The drawing under review shows one solid part. Ordinate dimensions are in mm from its lowest x, y, z. A direction names the side the tool comes from. Coordinates: 2 decimals unless noted, no trailing zeros. Write each loop counter-clockwise with the first axis right and the second up, starting at its lowest first coordinate (ties: lowest second). Pieces come first, ordered by that corner, then holes.
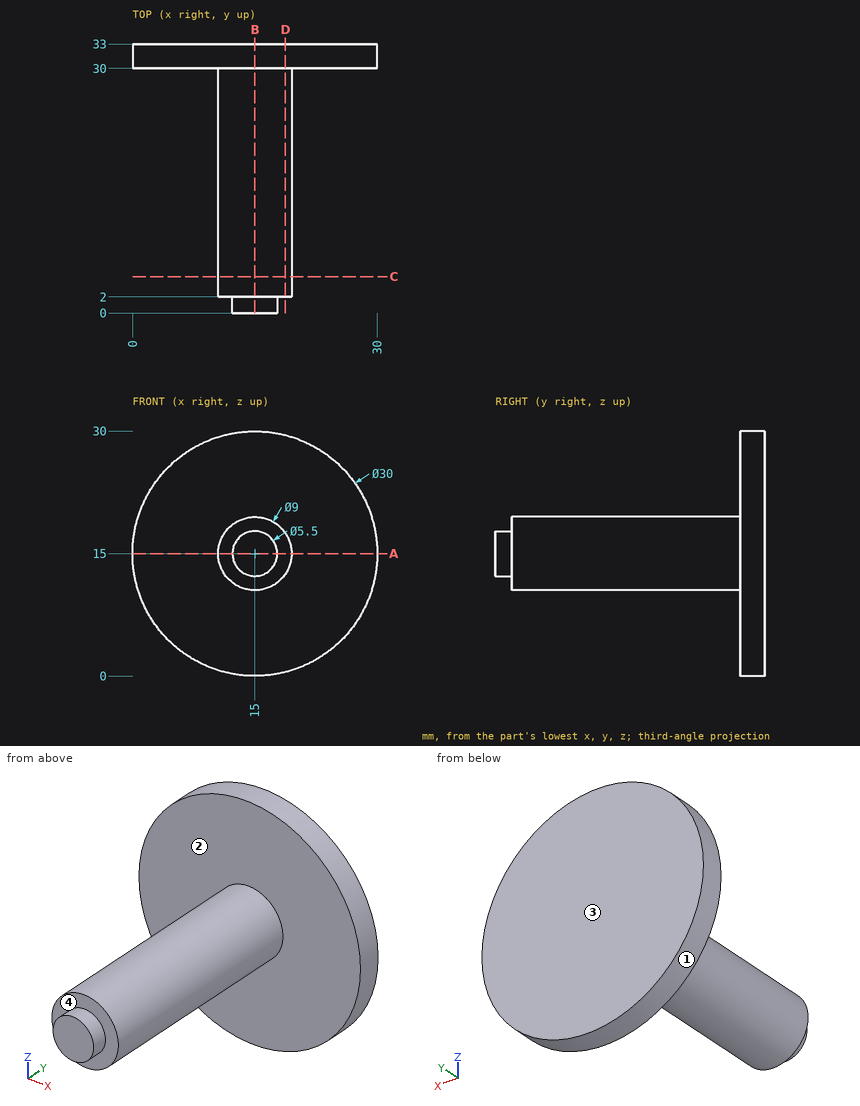
Q1. Draft analysis for pull direction Z (two halves, no side actions). For the marked faces 1 and 2, state which applies: +Z half, -Z half, draft (parallel to the pull), parting line (faces both ways), or undercut.
Ans:
face 1: parting line
face 2: draft
Q2. Add section D-D (x = 18.75). State the section outline as (y, z) points, then the cut area to 3 significant figures.
Ans:
outline: (2, 12.51) - (30, 12.51) - (30, 0.48) - (33, 0.48) - (33, 29.52) - (30, 29.52) - (30, 17.49) - (2, 17.49) - close
area: 226 mm2
Q3. Add section C-C (y = 4.5). State the section outline as (x, z) points.
Ans:
outline: circle Ø9 at (15, 15)
Q4. Add section A-A (z = 15). State the section outline as (x, y) points.
Ans:
outline: (0, 30) - (10.5, 30) - (10.5, 2) - (12.25, 2) - (12.25, 0) - (17.75, 0) - (17.75, 2) - (19.5, 2) - (19.5, 30) - (30, 30) - (30, 33) - (0, 33) - close
Q5. Clearance check with flat-ended pins moving along their axes: pin 1 Ø2 at (x, z) = (17, 22.5) entering from -Y; pin 2 Ø10 at (y, z) = (16, 11) entering from -X; pin 3 Ø10 at (x, y) = (20, 15.5) entering from +Z; pin 4 Ø2 at (x, y) = (9, 13.5) entering from -Z. State where each tip first meets the part, or that it passes through.
Ans:
pin 1: stops at y = 30
pin 2: stops at x = 10.5
pin 3: stops at z = 19.5
pin 4: passes through
Q6. Tool access review of the marked faces 3 and 4: name each direction out of +Z, -Z, +X, -X, +Y, -Y from which nothing blocks a thin tool from reaching the whole face with its end or side.
Ans:
face 3: +Z, -Z, +X, -X, +Y
face 4: -Y
Q7. Add section B-B (x = 15). State the section outline as (y, z) points, then the cut area to 3 significant figures.
Ans:
outline: (0, 12.25) - (2, 12.25) - (2, 10.5) - (30, 10.5) - (30, 0) - (33, 0) - (33, 30) - (30, 30) - (30, 19.5) - (2, 19.5) - (2, 17.75) - (0, 17.75) - close
area: 353 mm2
Q8. For probe 1 along X at (y, z) = (12.5, 15.25); probe 2 along Y at (x, z) = (18.5, 17.5); probe 3 along Y at (x, z) = (4, 14.5), list the stretches that pass through material, from the lowest coordinate up.
Ans:
probe 1: x = 10.51 to 19.49
probe 2: y = 2 to 33
probe 3: y = 30 to 33
